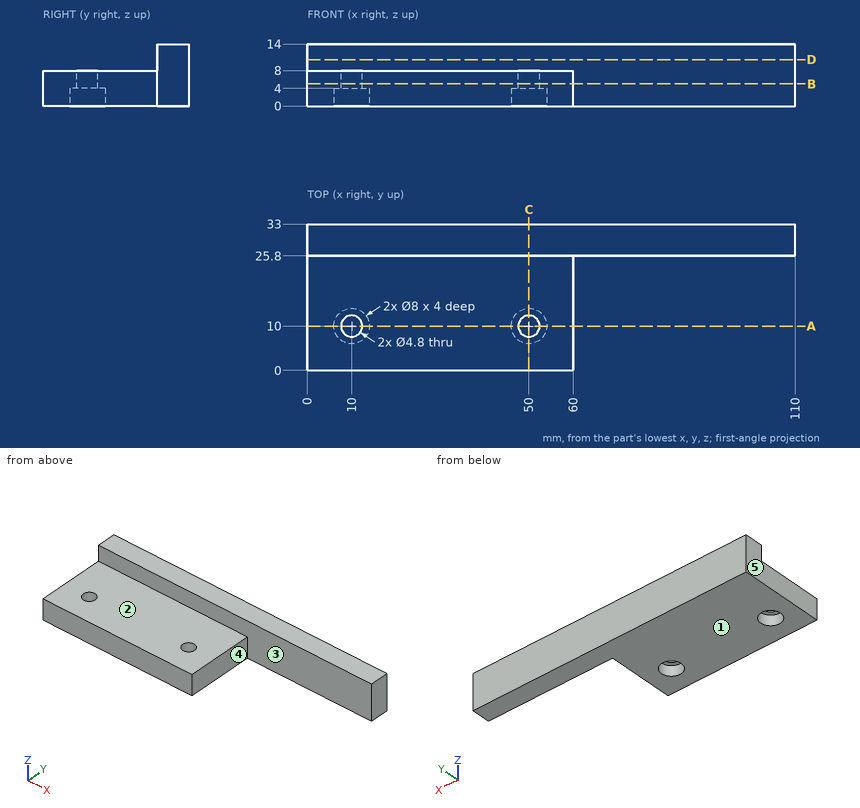
Print and shaded views of the part. All mm, measured from the part's lowest x, y and z. A direction names the side the tool comes from. Give positions to 0.01 mm unless a question says otherwise; leave off trailing zeros. Loops run counter-clockwise (first coordinate to the right, second up) from the corner with the lowest first, then second, coordinate; pieces in that order, holes last. Notation, with made-up numbers: (59.5, 58.25) - (63.5, 58.25) arc R21 ccw to (63.5, 94.25) - close; hole circle Ø2 at (65, 33.25). An arc over 180 degrees is marked (long way). One line per item, written item: value. Start each with the question number.
1. Slice it at D-D (z = 10.5). List the corners of the cut face in (x, y).
2. Slice it at A-A (y = 10). List the corners of the cut face in (x, z).
3. Slice it at C-C (x = 50). List the corners of the cut face in (y, z), plus the area to 3 significant figures.
4. Slice it at B-B (z = 5). List the corners of the cut face in (x, y), plus the area to 3 significant figures.
5. Which spindle directions (+Z, -Z, +X, -X, +Y, -Y) get a long thin tool onto all of the face, cutting with end or side? Do the marked faces 1, 2, 3, 4 and 5. Say none if no direction does.
6. Probe L1, parallel to Y at x = 10, z = 6.1; L2, parallel to Z at x = 41.5, y = 4.5; L3, parallel to Y at x = 99, z = 9. List the from-to ranges inside material, lowest first. Write a range as from..to.
7. Pin check, flat tips, straight feed: pin 1 (7.5 mm diameter, centred on x = 35.5, y = 14, fed in from +Z); pin 2 (4 mm diameter, centred on x = 10.5, y = 9, fed in from -Z); pin 3 (5 mm diameter, centred on y = 5.5, z = 7.5, fed in from +X). Stop position of each tip, or through.
Solution:
1. outline: (0, 25.8) - (110, 25.8) - (110, 33) - (0, 33) - close
2. outline: (0, 0) - (6, 0) - (6, 4) - (7.6, 4) - (7.6, 8) - (0, 8) - close; (12.4, 4) - (14, 4) - (14, 0) - (46, 0) - (46, 4) - (47.6, 4) - (47.6, 8) - (12.4, 8) - close; (52.4, 4) - (54, 4) - (54, 0) - (60, 0) - (60, 8) - (52.4, 8) - close
3. outline: (0, 0) - (6, 0) - (6, 4) - (7.6, 4) - (7.6, 8) - (0, 8) - close; (12.4, 4) - (14, 4) - (14, 0) - (33, 0) - (33, 14) - (25.8, 14) - (25.8, 8) - (12.4, 8) - close
3. area: 256 mm^2
4. outline: (0, 0) - (60, 0) - (60, 25.8) - (110, 25.8) - (110, 33) - (0, 33) - close; hole circle Ø4.8 at (10, 10); hole circle Ø4.8 at (50, 10)
4. area: 2,300 mm^2
5. face 1: -Z, +X, -X, +Y, -Y
5. face 2: +Z, +X, -X, -Y
5. face 3: +Z, +X, -Y
5. face 4: +Z, -Z, +X, -Y
5. face 5: +Z, -Z, -X, +Y, -Y
6. L1: y = 0..7.6, 12.4..33
6. L2: z = 0..8
6. L3: y = 25.8..33
7. pin 1: stops at z = 8
7. pin 2: stops at z = 4
7. pin 3: stops at x = 60
